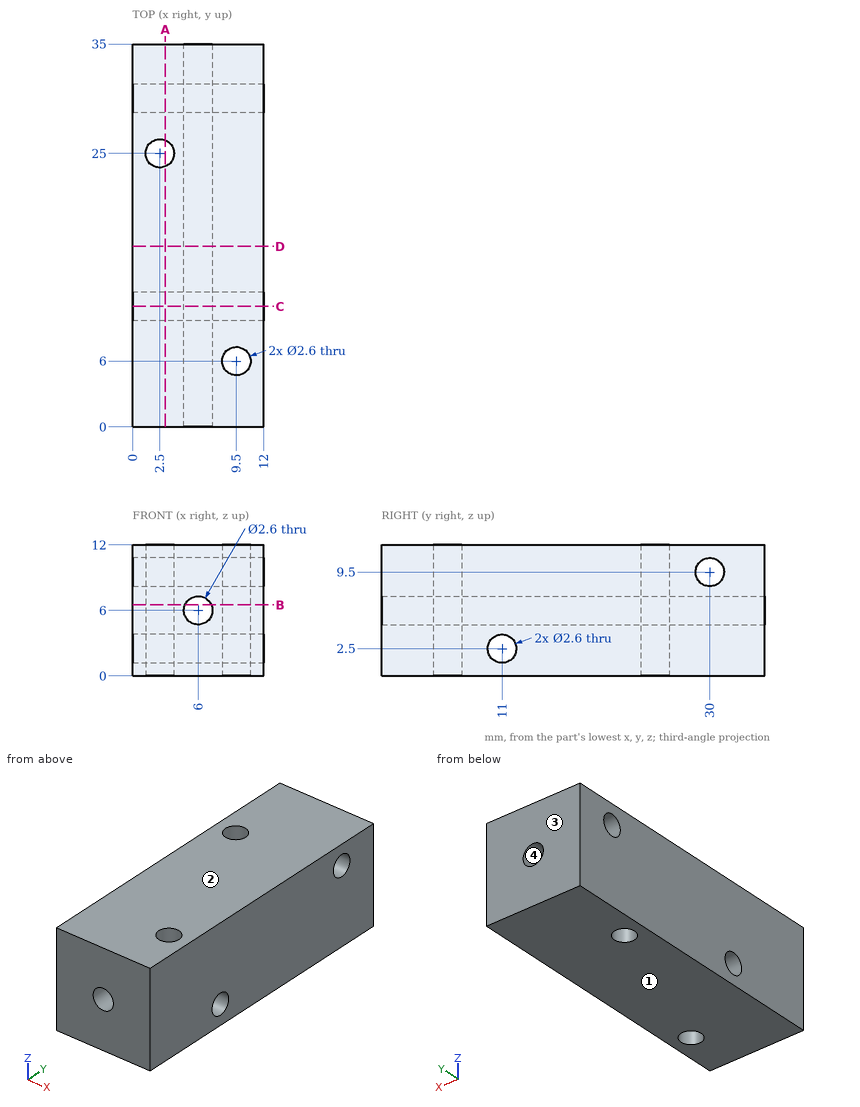
Check sheet for the drawn part. Datum: minimum x, y, z corner. Units: mm. Round coordinates to 2 decimals unless told otherwise and drop trailing zeros. Order: outer loops, then holes, each group sorted by start corner. A loop starts at its lowest first (then second) coordinate and runs counter-clockwise, first axis right, second up.
1. Section check A-A on x = 3. Record the cut outline in (y, z), then the cut area to 3 significant figures.
Final values:
outline: (0, 0) - (23.8, 0) - (23.8, 12) - (0, 12) - close; (26.2, 0) - (35, 0) - (35, 12) - (26.2, 12) - close; hole circle Ø2.6 at (11, 2.5); hole circle Ø2.6 at (30, 9.5)
area: 381 mm2
2. Section check C-C on y = 11. Record the cut outline in (x, z), then the cut area to 3 significant figures.
Final values:
outline: (0, 0) - (12, 0) - (12, 1.2) - (0, 1.2) - close; (0, 3.8) - (12, 3.8) - (12, 12) - (0, 12) - close; hole circle Ø2.6 at (6, 6)
area: 107 mm2
3. Section check B-B on z = 6.5. Record the cut outline in (x, y).
Final values:
outline: (0, 0) - (4.8, 0) - (4.8, 35) - (0, 35) - close; (7.2, 0) - (12, 0) - (12, 35) - (7.2, 35) - close; hole circle Ø2.6 at (2.5, 25); hole circle Ø2.6 at (9.5, 6)
4. Release check for a two-part mould opening along Z. For the marked faces 1, 2, 3 and 4 record: +Z half, -Z half, draft (parallel to the pull), parting line (faces both ways), or undercut.
Final values:
face 1: -Z half
face 2: +Z half
face 3: draft
face 4: undercut
5. Thickness scan on L1, parallel to Y at x = 9.5, z = 9.5; L2, parallel to X at y = 25, z = 4.5; L3, parallel to Z at x = 6, y = 9. Record the ranges inside material, lowest first.
Final values:
L1: y = 0 to 4.7, 7.3 to 28.7, 31.3 to 35
L2: x = 0 to 1.2, 3.8 to 12
L3: z = 0 to 4.7, 7.3 to 12
6. Section check D-D on y = 16.5. Record the cut outline in (x, z), then the cut area to 3 significant figures.
Final values:
outline: (0, 0) - (12, 0) - (12, 12) - (0, 12) - close; hole circle Ø2.6 at (6, 6)
area: 139 mm2
